Autodesk Inventor part; units mm, degrees
ref_plane "YZ Plane" through (0, 0, 0) normal (1, 0, 0) x (0, 1, 0)
ref_plane "XZ Plane" through (0, 0, 0) normal (0, 1, 0) x (-1, 0, 0)
ref_plane "XY Plane" through (0, 0, 0) normal (0, 0, 1) x (1, 0, 0)
sketch "Skizze1" plane through (0, 0, 0) normal (1, 0, 0) x (0, 1, 0)
  line L0 (0, 20) -> (0, -20)
  line L1 (0, 5) -> (2.5, 5)
  line L2 (2.5, 5) -> (2.5, 0)
  line L3 (2.5, 0) -> (0, 0) construction
  line L4 (2.5, 0) -> (4, 0)
  line L5 (4, 0) -> (4, -30)
  line L6 (4, -30) -> (0, -30)
  line L7 (2.5, -8) -> (2.5, -30)
  line L8 (1, 5) -> (1, -8)
  line L9 (1, -8) -> (2.5, -8)
  dimension "d0" = 40
  dimension "d1" = 5
  dimension "d2" = 5
  dimension "d4" = 8
  dimension "d5" = 30
  dimension "d8" = 22
  dimension "d9" = 5
  dimension "d10" = 2
revolve "Umdrehung1" add sketch "Skizze1" angle 360 about axis through (0, 0, 20) along (0, 0, -1)
sketch "Skizze2" plane through (0, 0, 0) normal (0, 1, 0) x (-1, 0, 0)
  line L0 (-4, -30) -> (4, -30)
  line L1 (-4, 0) -> (4, 0)
  point P0 (0, 0)
  point P1 (0, -5)
  point P2 (0, -18)
  dimension "d12" = 12
  dimension "d13" = 5
hole "Bohrung1" at (0, 0, -5) direction (0, 1, 0) diameter 2 end through all
hole "Bohrung2" at (0, 0, -18) direction (0, 1, 0) diameter 3 end through all
thread "Gewinde1"
thread "Gewinde2"
chamfer "Fase1" distance 0.25 angle 45 2 edges at (1.5, 3.7081, -18.0006) (-1.5, 3.7081, -17.9994)
chamfer "Fase2" distance 0.25 angle 45 2 edges at (1, 3.873, -4.9999) (-1, 3.873, -5.0001)
chamfer "Fase3" distance 0.25 angle 45 1 edges at (0, -1, 5)
chamfer "Fase4" distance 0.25 angle 45 1 edges at (0, -2.5, -30)
chamfer "Fase5" distance 0.25 angle 45 1 edges at (0, -2.5, 5)
chamfer "Fase6" distance 0.25 angle 45 1 edges at (0, -4, 0)
chamfer "Fase7" distance 0.25 angle 45 1 edges at (0, -4, -30)
properties part number "BT802_goteln20_21_Zeichenmaschine_Welle_2zu5"
Here's how the part is built. I have some questions about the finished solid (model axes, mm). A direction names the side the tool comes from. Round coordinates to 2 decimals unless told otherwise and drop trailing zeros. Write each loop counter-clockwise with the first axis right and the second up, starting at its lowest first coordinate (ties: lowest second). Pieces come first, ordered by that corner, then holes. Notation, with made-up numbers: M -38.75,69.25 L 13.25,69.25 A8 cw 13.25,84.25 Z; hole C 51.5,23.5 d5. An arc over 180 degrees is marked long. Answer as CSV lines item,"result". Start each with the question number.
1. Suppose I cut it at B-B on z = 3.5. Write out the boundary of the cut face in (x, y), then the cut area to 3 significant figures.
2. On a 3-axis mill with a long thin cutter (end or side, diameter ignored), from which of +Z, -Z, +X, -X, +Y, -Y can I reach the whole of each face in a straight line? I mean faces 1 (the cylindrical face through (0, -1, -2)), 2 (the flat face through (3, 0, 0)), 3 (the cylindrical face through (0.575, 2.887, -19.386)), 4 (the flat face through (-1, 1, 5)), 5 (the flat face through (-1, 1, -8)). Say none if no direction works.
3. I need wall thicknesses on probe 1 along Z at (x, y) = (0.75, 3.5); probe 2 along X at (y, z) = (0, -1.5); probe 3 along X at (y, z) = (0.75, -14). Which ranges of each line are inside material? Lowest first, please.
4. Thinking about a two-plate mould opening in X: for faces 6 (the flat face through (3, -1, -30)), 7 (the cylindrical face through (0, -4, -15)), 8 (the cylindrical face through (0, 2, -6)), which applies, released by +X, released by -X, zero draft, split by the parting line, or undercut?
5. I'm going to push a flat-ended pin straight in: pin 1 Ø3 at (x, y) = (0, 0) entering from -Z. Where does the tip first touch, or does it pass through?
6. Suppose I cut it at A-A on z = -25. Write out the boundary of the cut face in (x, y).
Check result:
1,outline,"C 0,0 d5; hole C 0,0 d2"
1,area,"16.5 mm2"
2,face 1,"+Z, -Z"
2,face 2,"+Z"
2,face 3,"+Y"
2,face 4,"+Z, +X, -X, +Y, -Y"
2,face 5,"-Z"
3,probe 1,"z = -30 to -19.3, -16.7 to -5.66, -4.34 to 0"
3,probe 2,"x = -4 to -1, 1 to 4"
3,probe 3,"x = -3.93 to -2.38, 2.38 to 3.93"
4,face 6,"zero draft"
4,face 7,"split by the parting line"
4,face 8,"undercut"
5,pin 1,"stops at z = -8"
6,outline,"C 0,0 d8; hole C 0,0 d5"
